Design review of the part built by this model. Coordinates are the model's own, in mm. A direction names the side the tool comes from. Round coordinates to 2 decimals unless told otherwise and drop trailing zeros. Order: outer loops, then holes, each group sorted by start corner. A loop starts at its lowest first (then second) coordinate and runs counter-clockwise, first axis right, second up. Notation, with made-up numbers: (-28.75, -8) - (8.25, -8) arc R5 cw to (8.25, -4) - close; hole circle Ø11 at (1.25, 69.5). An arc over 180 degrees is marked (long way). Write item = value, one per line.
from build123d import *

# Parameters (mm, degrees)
CROQUIS1_W              = 80.5
CROQUIS1_H              = 53.3
SALIENTE_EXTRUIR1_DEPTH = 5
CROQUIS2_W              = 96
CROQUIS2_H              = 64.811604732
SALIENTE_EXTRUIR2_DEPTH = 4
CROQUIS3_W              = 10
CROQUIS3_H              = 15
CORTAR_EXTRUIR1_DEPTH   = 6.8
CROQUIS4_W              = 5.8
CROQUIS4_H              = 2.5
CROQUIS4_W_2            = 2.7
SALIENTE_EXTRUIR3_DEPTH = 7
CROQUIS5_W              = 70
CROQUIS5_H              = 35
CORTAR_EXTRUIR2_DEPTH   = 5


with BuildPart() as part:
    # Croquis1 → Saliente-Extruir1 (new body)
    with BuildSketch(Plane.XY):
        Polygon((-43.45, 24), (-40.25, 24), (-40.25, 29.3), (-48, 29.3), (-48, -35.511604732), (48, -35.511604732), (48, 29.3), (40.25, 29.3), (40.25, 24), (43.45, 24), (43.45, -30.7), (-43.45, -30.7), align=None)
        with Locations((0, 2.65)):
            Rectangle(CROQUIS1_W, CROQUIS1_H)
    extrude(amount=SALIENTE_EXTRUIR1_DEPTH)

    # Croquis2 → Saliente-Extruir2 (add)
    with BuildSketch(Plane.XY.offset(5)):
        with Locations((0, -3.105802366)):
            Rectangle(CROQUIS2_W, CROQUIS2_H)
    extrude(amount=SALIENTE_EXTRUIR2_DEPTH)

    # Croquis3 → Cortar-Extruir1 (cut)
    with BuildSketch(Plane(origin=(0, 0, 0), x_dir=(-1, 0, 0), z_dir=(0, 0, -1))):
        with Locations((12.95, -31.5)):
            Rectangle(CROQUIS3_W, CROQUIS3_H)
    extrude(amount=-CORTAR_EXTRUIR1_DEPTH, mode=Mode.SUBTRACT)

    # Croquis4 → Saliente-Extruir3 (add)
    with BuildSketch(Plane(origin=(0, 0, 0), x_dir=(-1, 0, 0), z_dir=(0, 0, -1))):
        with Locations((40.55, -29.45)):
            Rectangle(CROQUIS4_W, CROQUIS4_H)
        with Locations((-42.1, -29.45)):
            Rectangle(CROQUIS4_W_2, CROQUIS4_H)
    extrude(amount=-SALIENTE_EXTRUIR3_DEPTH)

    # Croquis5 → Cortar-Extruir2 (cut)
    with BuildSketch(Plane(origin=(0, 0, 0), x_dir=(-1, 0, 0), z_dir=(0, 0, -1))):
        Rectangle(CROQUIS5_W, CROQUIS5_H)
    extrude(amount=-CORTAR_EXTRUIR2_DEPTH, mode=Mode.SUBTRACT)


solid = part.part
1) To check wall thickness, follow L1, parallel to Y at x = 32, z = 1.5; L2, parallel to X at y = 0, z = 4; L3, parallel to X at y = -21, z = 3.25. State the ranges of each line that lie inside material, in increasing order. Write a range as from..to.
Findings:
L1 = -35.51..-30.7, -24..-17.5, 17.5..29.3
L2 = -48..-43.45, -40.25..-35, 35..40.25, 43.45..48
L3 = -48..-43.45, -40.25..40.25, 43.45..48
2) We need section C-C on y = 22.5. Write out the cut boundary in (x, z), and give its area (3 significant figures).
Findings:
outline = (-48, 0) - (-43.45, 0) - (-43.45, 5) - (-40.25, 5) - (-40.25, 0) - (40.25, 0) - (40.25, 5) - (43.45, 5) - (43.45, 0) - (48, 0) - (48, 9) - (-48, 9) - close
area = 832 mm^2
3) Clearance check with a flat-ended pin moving along its axis: pin 1 Ø17.5 at (x, y) = (15, 2) entering from -Z. State where the tip first meets the part, or that it passes through.
Findings:
pin_1 = 5
4) The part is to be moulded in two halves that separate along X. For faces 1 (the flat face through (-48, -4, 4)), 2 (the flat face through (-1, -3, 9)), 3 (the flat face through (-28, -30.7, 2)), say which applies: released by +X, released by -X, zero draft, split by the parting line, or undercut.
Findings:
face_1 = released by -X
face_2 = zero draft
face_3 = undercut
5) We need section A-A on z = 2.5. Write out the cut boundary in (x, y), and give its area (3 significant figures).
Findings:
outline = (-48, -35.51) - (-17.95, -35.51) - (-17.95, -30.7) - (-37.65, -30.7) - (-37.65, -28.2) - (-43.45, -28.2) - (-43.45, 24) - (-40.25, 24) - (-40.25, -24) - (40.25, -24) - (40.25, 24) - (43.45, 24) - (43.45, -28.2) - (40.75, -28.2) - (40.75, -30.7) - (-7.95, -30.7) - (-7.95, -35.51) - (48, -35.51) - (48, 29.3) - (-48, 29.3) - close; hole (-35, -17.5) - (35, -17.5) - (35, 17.5) - (-35, 17.5) - close
area = 2,860 mm^2
6) We need section B-B on x = -36.5. Write out the cut boundary in (y, z), and give its area (3 significant figures).
Findings:
outline = (-35.51, 0) - (-30.7, 0) - (-30.7, 5) - (-24, 5) - (-24, 0) - (29.3, 0) - (29.3, 9) - (-35.51, 9) - close
area = 550 mm^2
7) For faces 4 (the flat face through (-7.95, -32, 4)), 5 (the flat face through (43.45, -2, 2)), 6 (the flat face through (0, -20, 0)), list the 3-axis set-ups (+Z, -Z, +X, -X, +Y, -Y) from which the entire face can be reached by the end or side of a thin tool; tool diameter is ignored.
Findings:
face_4 = -Z, -Y
face_5 = -Z
face_6 = -Z, +X, -X, +Y, -Y
8) We need section D-D on y = 2.5. Write out the cut boundary in (x, z), and give its area (3 significant figures).
Findings:
outline = (-48, 0) - (-43.45, 0) - (-43.45, 5) - (-40.25, 5) - (-40.25, 0) - (-35, 0) - (-35, 5) - (35, 5) - (35, 0) - (40.25, 0) - (40.25, 5) - (43.45, 5) - (43.45, 0) - (48, 0) - (48, 9) - (-48, 9) - close
area = 482 mm^2
